Check sheet for the drawn part. Datum: minimum x, y, z corner. Units: mm. Coordinates: 2 decimals unless noted, no trailing zeros. Write each loop counter-clockwise with the first axis right and the second up, starting at its lowest first coordinate (ties: lowest second). Pieces come first, ordered by that corner, then holes. Notation, with made-up numbers: (-12.5, 53) - (2.5, 53) arc R10 cw to (2.5, 59) - close; hole circle Ø4 at (-38, 24). An arc over 180 degrees is marked (long way). Use CSV: the item, a comma, the result in double quotes. Start each with the question number.
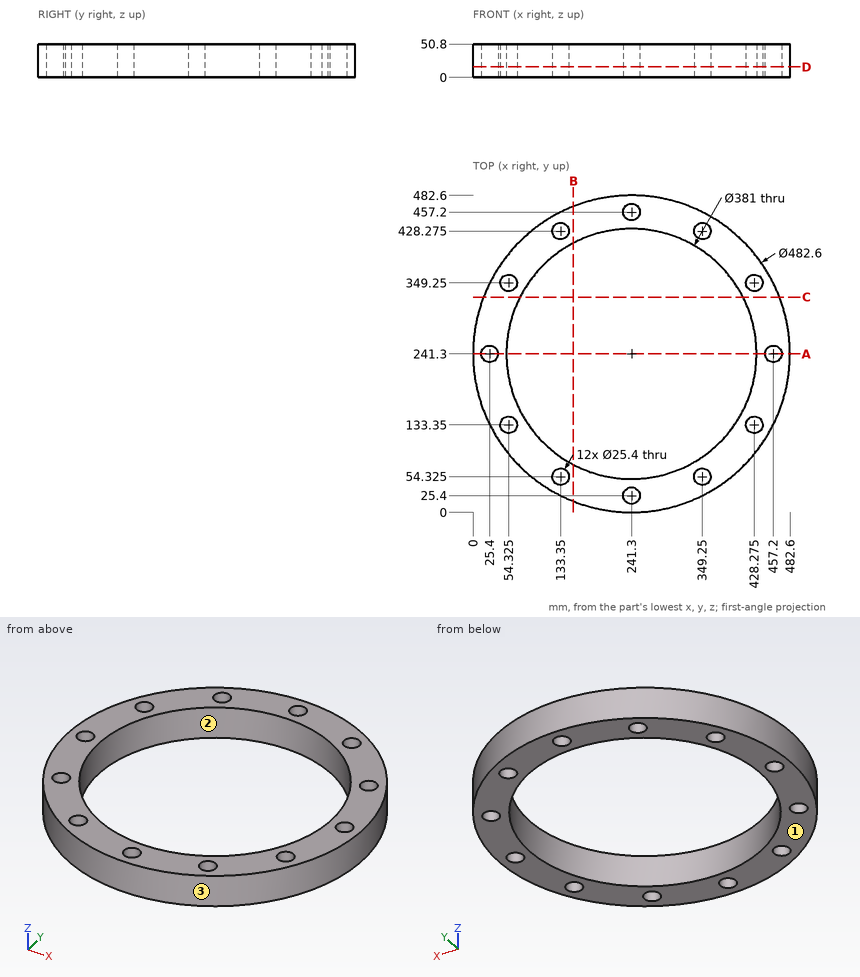
Q1. Cross-section at D-D (z = 16). State how many separate pieces and enclosed holes the cut face has, plus the area to 3 significant figures.
Q2. Cross-section at C-C (y = 327.5). Record the cut outline in (x, z).
Q3. Release check for a two-part mould opening along X. For the marked faces 1, 2 and 3 record: released by +X, released by -X, zero draft, split by the parting line, or undercut.
Q4. Gauge pin test, flat ends, axial feed: pin 1 (15 mm diameter, centred on x = 133.35, y = 54.33, fed in from -Z); pin 2 (6 mm diameter, centred on y = 259.5, z = 21, fed in from +X); pin 3 (3 mm diameter, centred on x = 215, z = 38.5, fed in from -Y); pin 4 (3 mm diameter, centred on x = 425.5, z = 20, fed in from -Y). Record the tip position at first contact, or that the pin passes through.
Q5. Cross-section at B-B (x = 153). Record the cut outline in (y, z), plus the area to 3 significant figures.
Q6. Scan lines: line 1 along X through (y, z) = (240, 38.5); line 2 along Y through (x, z) = (338, 46.5); line 3 along Y through (x, z) = (349.25, 34.5) (1 decimal). Record each from-to range of solid material in increasing order. Write a range as from..to.
Q7. Cross-section at A-A (y = 241.3). Record the cut outline in (x, z).
Reply:
1,separate pieces,"1"
1,enclosed holes,"13"
1,area,"62,800 mm^2"
2,outline,"(15.92, 0) - (71.42, 0) - (71.42, 50.8) - (15.92, 50.8) - close; (411.18, 0) - (466.68, 0) - (466.68, 50.8) - (411.18, 50.8) - close"
3,face 1,"zero draft"
3,face 2,"undercut"
3,face 3,"split by the parting line"
4,pin 1,"through"
4,pin 2,"x = 482.12"
4,pin 3,"y = 1.28"
4,pin 4,"y = 83.67"
5,outline,"(16.74, 0) - (72.5, 0) - (72.5, 50.8) - (16.74, 50.8) - close; (410.1, 0) - (465.86, 0) - (465.86, 50.8) - (410.1, 50.8) - close"
5,area,"5,670 mm^2"
6,line 1,"0..12.77, 38.03..50.8, 431.8..444.57, 469.83..482.6"
6,line 2,"20.22..48.43, 60.22..77.17, 405.43..422.38, 434.17..462.38"
6,line 3,"25.5..41.6, 67..84.3, 398.3..415.6, 441..457.1"
7,outline,"(0, 0) - (12.7, 0) - (12.7, 50.8) - (0, 50.8) - close; (38.1, 0) - (50.8, 0) - (50.8, 50.8) - (38.1, 50.8) - close; (431.8, 0) - (444.5, 0) - (444.5, 50.8) - (431.8, 50.8) - close; (469.9, 0) - (482.6, 0) - (482.6, 50.8) - (469.9, 50.8) - close"
